```python
from build123d import *

# Parameters (mm, degrees)
SKETCH1_W           = 75
SKETCH1_H           = 60
SKETCH1_R           = 2.2
BOSS_EXTRUDE1_DEPTH = 11
SKETCH2_W           = 60
SKETCH2_H           = 241
BOSS_EXTRUDE2_DEPTH = 8
SKETCH4_W           = 75
SKETCH4_H           = 6
BOSS_EXTRUDE3_DEPTH = 150
CUT_EXTRUDE1_DEPTH  = 28
SKETCH6_R           = 3.2
CUT_EXTRUDE2_DEPTH  = 8


with BuildPart() as part:
    # Sketch1 → Boss-Extrude1 (new body)
    with BuildSketch(Plane(origin=(0, 0, 0), x_dir=(1, 0, 0), z_dir=(0, 1, 0))):
        Rectangle(SKETCH1_W, SKETCH1_H)
        with Locations(Location((-7.5, 25, 0), (0, 0, 270))):
            Circle(SKETCH1_R, mode=Mode.SUBTRACT)
        with Locations(Location((-7.5, -25, 0), (0, 0, 270))):
            Circle(SKETCH1_R, mode=Mode.SUBTRACT)
        with Locations(Location((17.5, 25, 0), (0, 0, 270))):
            Circle(SKETCH1_R, mode=Mode.SUBTRACT)
        with Locations(Location((17.5, 0, 0), (0, 0, 270))):
            Circle(SKETCH1_R, mode=Mode.SUBTRACT)
        with Locations(Location((17.5, -25, 0), (0, 0, 270))):
            Circle(SKETCH1_R, mode=Mode.SUBTRACT)
        with Locations(Location((-32.5, 25, 0), (0, 0, 270))):
            Circle(SKETCH1_R, mode=Mode.SUBTRACT)
        with Locations(Location((-32.5, 0, 0), (0, 0, 270))):
            Circle(SKETCH1_R, mode=Mode.SUBTRACT)
        with Locations(Location((-32.5, -25, 0), (0, 0, 270))):
            Circle(SKETCH1_R, mode=Mode.SUBTRACT)
        with Locations(Location((-7.5, 0, 0), (0, 0, 270))):
            Circle(SKETCH1_R, mode=Mode.SUBTRACT)
    extrude(amount=BOSS_EXTRUDE1_DEPTH)

    # Sketch2 → Boss-Extrude2 (add)
    with BuildSketch(Plane(origin=(37.5, 0, 0), x_dir=(0, 0, -1), z_dir=(1, 0, 0))):
        with Locations((0, 60.5)):
            Rectangle(SKETCH2_W, SKETCH2_H)
    extrude(amount=BOSS_EXTRUDE2_DEPTH)

    # Sketch4 → Boss-Extrude3 (add)
    with BuildSketch(Plane(origin=(0, 11, 0), x_dir=(1, 0, 0), z_dir=(0, 1, 0))):
        with Locations((0, 11)):
            Rectangle(SKETCH4_W, SKETCH4_H)
        with Locations((0, -11)):
            Rectangle(SKETCH4_W, SKETCH4_H)
    extrude(amount=BOSS_EXTRUDE3_DEPTH)

    # Sketch5 → Cut-Extrude1 (cut)
    with BuildSketch(Plane.XY.offset(14)):
        Polygon((37.5, 161), (-37.5, 161), (-37.5, 11), align=None)
    extrude(amount=-CUT_EXTRUDE1_DEPTH, mode=Mode.SUBTRACT)

    # Sketch6 → Cut-Extrude2 (cut)
    with BuildSketch(Plane(origin=(45.5, 0, 0), x_dir=(0, 0, -1), z_dir=(1, 0, 0))):
        with Locations((-20, 173)):
            Circle(SKETCH6_R)
        with Locations((0, 173)):
            Circle(SKETCH6_R)
        with Locations((20, 173)):
            Circle(SKETCH6_R)
        with Locations((0, 158)):
            Circle(SKETCH6_R)
        with Locations((-20, 158)):
            Circle(SKETCH6_R)
        with Locations((20, 158)):
            Circle(SKETCH6_R)
        with Locations((-20, 143)):
            Circle(SKETCH6_R)
        with Locations((0, 143)):
            Circle(SKETCH6_R)
        with Locations((20, 143)):
            Circle(SKETCH6_R)
        with Locations((-20, 128)):
            Circle(SKETCH6_R)
        with Locations((0, 128)):
            Circle(SKETCH6_R)
        with Locations((20, 128)):
            Circle(SKETCH6_R)
        with Locations((-20, 113)):
            Circle(SKETCH6_R)
        with Locations((0, 113)):
            Circle(SKETCH6_R)
        with Locations((20, 113)):
            Circle(SKETCH6_R)
        with Locations((20, 98)):
            Circle(SKETCH6_R)
        with Locations((0, 98)):
            Circle(SKETCH6_R)
        with Locations((-20, 98)):
            Circle(SKETCH6_R)
        with Locations((-20, 83)):
            Circle(SKETCH6_R)
        with Locations((0, 83)):
            Circle(SKETCH6_R)
        with Locations((20, 83)):
            Circle(SKETCH6_R)
        with Locations((20, 68)):
            Circle(SKETCH6_R)
        with Locations((0, 68)):
            Circle(SKETCH6_R)
        with Locations((-20, 68)):
            Circle(SKETCH6_R)
        with Locations((-20, 53)):
            Circle(SKETCH6_R)
        with Locations((0, 53)):
            Circle(SKETCH6_R)
        with Locations((20, 53)):
            Circle(SKETCH6_R)
        with Locations((20, 38)):
            Circle(SKETCH6_R)
        with Locations((0, 38)):
            Circle(SKETCH6_R)
        with Locations((-20, 38)):
            Circle(SKETCH6_R)
        with Locations((-20, 23)):
            Circle(SKETCH6_R)
        with Locations((0, 23)):
            Circle(SKETCH6_R)
        with Locations((20, 23)):
            Circle(SKETCH6_R)
        with Locations((20, 8)):
            Circle(SKETCH6_R)
        with Locations((-20, 8)):
            Circle(SKETCH6_R)
        with Locations((0, 8)):
            Circle(SKETCH6_R)
        with Locations((-20, -7)):
            Circle(SKETCH6_R)
        with Locations((0, -7)):
            Circle(SKETCH6_R)
        with Locations((20, -7)):
            Circle(SKETCH6_R)
        with Locations((20, -22)):
            Circle(SKETCH6_R)
        with Locations((0, -22)):
            Circle(SKETCH6_R)
        with Locations((-20, -22)):
            Circle(SKETCH6_R)
        with Locations((-20, -37)):
            Circle(SKETCH6_R)
        with Locations((0, -37)):
            Circle(SKETCH6_R)
        with Locations((20, -37)):
            Circle(SKETCH6_R)
        with Locations((20, -52)):
            Circle(SKETCH6_R)
        with Locations((0, -52)):
            Circle(SKETCH6_R)
        with Locations((-20, -52)):
            Circle(SKETCH6_R)
    extrude(amount=-CUT_EXTRUDE2_DEPTH, mode=Mode.SUBTRACT)


solid = part.part
```
Input: part model. Units: mm. Frame: model coordinates. A direction names the side the tool comes from. Give positions to 0.01 mm unless a question says otherwise; leave off trailing zeros. Order: outer loops, then holes, each group sorted by start corner. A loop starts at its lowest first (then second) coordinate and runs counter-clockwise, first axis right, second up. Notation, with made-up numbers: (-40, 76.5) - (5, 76.5) arc R26 cw to (5, 105.5) - close; hole circle Ø11 at (34.25, -5.5). An arc over 180 degrees is marked (long way). Use a Markdown table: item, result.
(1) Section query A-A (y = 23). Output: boundary loops of the cut face in (x, z).
Computed values:
| item | result |
|---|---|
| outline | (-31.5, -14) - (37.5, -14) - (37.5, -16.8) - (45.5, -16.8) - (45.5, -3.2) - (37.5, -3.2) - (37.5, -8) - (-31.5, -8) - close; (-31.5, 8) - (37.5, 8) - (37.5, 3.2) - (45.5, 3.2) - (45.5, 16.8) - (37.5, 16.8) - (37.5, 14) - (-31.5, 14) - close; (37.5, -30) - (45.5, -30) - (45.5, -23.2) - (37.5, -23.2) - close; (37.5, 23.2) - (45.5, 23.2) - (45.5, 30) - (37.5, 30) - close |
(2) Draft query along Z for faces 1 (the flat face through (16, 52, -14)), 2 (the flat face through (-1, 11, -22)), 3 (the cylindrical face through (41.556, -23.947, -17.461)). Return one class per face: released by +Z, released by -Z, zero draft, split by the parting line, or undercut.
Computed values:
| item | result |
|---|---|
| face 1 | released by -Z |
| face 2 | zero draft |
| face 3 | undercut |
(3) Section query C-C (z = 10.5). Output: boundary loops of the cut face in (x, y), then the cut area to 3 significant figures.
Computed values:
| item | result |
|---|---|
| outline | (-37.5, 0) - (37.5, 0) - (37.5, -60) - (45.5, -60) - (45.5, 181) - (37.5, 181) - (37.5, 161) - (-37.5, 11) - close |
| area | 8,380 mm2 |
(4) Section query B-B (x = -7.5). Output: boundary loops of the cut face in (y, z), then the cut area to 3 significant figures.
Computed values:
| item | result |
|---|---|
| outline | (0, -30) - (11, -30) - (11, -27.2) - (0, -27.2) - close; (0, -22.8) - (11, -22.8) - (11, -14) - (71, -14) - (71, -8) - (11, -8) - (11, -2.2) - (0, -2.2) - close; (0, 2.2) - (11, 2.2) - (11, 8) - (71, 8) - (71, 14) - (11, 14) - (11, 22.8) - (0, 22.8) - close; (0, 27.2) - (11, 27.2) - (11, 30) - (0, 30) - close |
| area | 1,230 mm2 |
(5) Section query D-D (y = -22). Output: boundary loops of the cut face in (x, z).
Computed values:
| item | result |
|---|---|
| outline | (37.5, -30) - (45.5, -30) - (45.5, -23.2) - (37.5, -23.2) - close; (37.5, -16.8) - (45.5, -16.8) - (45.5, -3.2) - (37.5, -3.2) - close; (37.5, 3.2) - (45.5, 3.2) - (45.5, 16.8) - (37.5, 16.8) - close; (37.5, 23.2) - (45.5, 23.2) - (45.5, 30) - (37.5, 30) - close |
(6) Pin query (flat end, axial travel): pin 1 (1 mm diameter, centred on x = -16.5, z = 14, fed in from +Y); pin 2 (7.5 mm diameter, centred on y = 128, z = 20, fed in from +X); pin 3 (5 mm diameter, centred on y = -22, z = -20, fed in from +X); pin 4 (7.5 mm diameter, centred on y = 38, z = 0, fed in from -X). Return the tip coordinate at first contact, or that it passes through.
Computed values:
| item | result |
|---|---|
| pin 1 | stops at y = 54 |
| pin 2 | stops at x = 45.5 |
| pin 3 | passes through |
| pin 4 | stops at x = 37.5 |
(7) Line query: line 1 (X direction, y = 4, z = -25); line 2 (Z direction, x = 42, y = 128); line 3 (Z direction, x = -4.5, y = 16). Output: solid intervals per line, ascending. Write a range as from..to.
Computed values:
| item | result |
|---|---|
| line 1 | x = -37.5..-34.7, -30.3..-9.7, -5.3..15.3, 19.7..45.5 |
| line 2 | z = -30..-23.2, -16.8..-3.2, 3.2..16.8, 23.2..30 |
| line 3 | z = -14..-8, 8..14 |
(8) Access query for faces 4 (the cylindrical face through (-5.32, 5.42, -0.29)), 5 (the flat face through (-1, 11, 0)), 6 (the cylindrical face through (41.6, 8.1, -16.8)). Directions: +Z, -Z, +X, -X, +Y, -Y. A direction counts if a zero-diameter tool reaches every point of the face in a straight line with its end or side. Return the directions, or none.
Computed values:
| item | result |
|---|---|
| face 4 | +Y, -Y |
| face 5 | -X, +Y |
| face 6 | +X |
